```python
from build123d import *

# Parameters (mm, degrees)
SKETCH1_R           = 4.1275
BOSS_EXTRUDE2_DEPTH = 9.525
SKETCH3_R           = 6.35
CUT_EXTRUDE1_DEPTH  = 3.81
SKETCH4_W           = 33.423596482
SKETCH4_H           = 7.62
CUT_EXTRUDE3_DEPTH  = 53.073871807
FILLET3_R           = 0.8128
CHAMFER5_SIZE       = 0.8128


with BuildPart() as part:
    # Sketch1 → Boss-Extrude2 (new, symmetric)
    with BuildSketch(Plane.XY):
        with BuildLine():
            Line((0, 12.7), (31.75, 12.7))
            ThreePointArc((31.75, 12.7), (44.45, 0), (31.75, -12.7))
            Line((31.75, -12.7), (0, -12.7))
            ThreePointArc((0, -12.7), (-12.7, 0), (0, 12.7))
        make_face()
        with Locations(Location((0, 0, 0), (0, 0, 180))):
            Circle(SKETCH1_R, mode=Mode.SUBTRACT)
        with Locations(Location((31.75, 0, 0), (0, 0, 180))):
            Circle(SKETCH1_R, mode=Mode.SUBTRACT)
    extrude(amount=BOSS_EXTRUDE2_DEPTH, both=True)

    # Sketch3 → Cut-Extrude1 (cut)
    with BuildSketch(Plane.XY.offset(9.525)):
        Circle(SKETCH3_R)
        with Locations((31.75, 0)):
            Circle(SKETCH3_R)
    cut_extrude1 = extrude(amount=-CUT_EXTRUDE1_DEPTH, mode=Mode.SUBTRACT)

    # Mirror1: Cut-Extrude1 across plane
    add(cut_extrude1.mirror(Plane.XY), mode=Mode.SUBTRACT)

    # Sketch4 → Cut-Extrude3 (cut, through all)
    with BuildSketch(Plane(origin=(0, 12.7, 0), x_dir=(1, 0, 0), z_dir=(0, 1, 0))):
        with Locations((35.707937548, 0)):
            Rectangle(SKETCH4_W, SKETCH4_H)
        with Locations((-3.957937548, 0)):
            Rectangle(SKETCH4_W, SKETCH4_H)
    extrude(amount=-CUT_EXTRUDE3_DEPTH, mode=Mode.SUBTRACT)

    # Fillet3
    fillet3_edges = [part.edges().sort_by_distance(p)[0] for p in [
        (44.45, 0, 9.525),
        (15.875, 12.7, 9.525),
        (-12.7, 0, 9.525),
        (15.875, 12.7, -9.525),
        (25.373069653, 12.7, -3.81),
        (6.376930347, 12.7, 3.81),
        (44.45, 0, -9.525),
        (15.875, -12.7, -9.525),
        (-12.7, 0, -9.525),
        (6.376930347, -12.7, -3.81),
        (-12.7, 0, -3.81),
        (-12.7, 0, 3.81),
        (6.376930347, -12.7, 3.81),
        (12.753860693, -12.7, 0),
        (12.753860693, 12.7, 0),
        (6.376930347, 12.7, -3.81),
        (25.373069653, 12.7, 3.81),
        (18.996139307, 12.7, 0),
        (44.45, 0, -3.81),
        (25.373069653, -12.7, -3.81),
        (25.373069653, -12.7, 3.81),
        (44.45, 0, 3.81),
        (15.875, -12.7, 9.525),
        (18.996139307, -12.7, 0),
    ]]
    fillet(fillet3_edges, radius=FILLET3_R)

    # Chamfer5
    chamfer5_edges = [part.edges().sort_by_distance(p)[0] for p in [
        (4.1275, 0, 5.715),
        (-6.35, 0, 9.525),
        (35.8775, 0, 5.715),
        (25.4, 0, 9.525),
        (-6.35, 0, -9.525),
        (4.1275, 0, -5.715),
        (25.4, 0, -9.525),
        (35.8775, 0, -5.715),
        (4.1275, 0, -3.81),
        (4.1275, 0, 3.81),
        (35.8775, 0, -3.81),
        (35.8775, 0, 3.81),
    ]]
    chamfer(chamfer5_edges, length=CHAMFER5_SIZE)


solid = part.part
```
CAD build for the part. Positions are in the model's coordinates, mm. A direction names the side the tool comes from. Round coordinates to 2 decimals unless told otherwise and drop trailing zeros. Write each loop counter-clockwise with the first axis right and the second up, starting at its lowest first coordinate (ties: lowest second). Pieces come first, ordered by that corner, then holes. Notation, with made-up numbers: (50, -8) -> (66, -8) arc R26 cw to (66, 8) -> close; hole circle Ø8 at (30.5, -21). An arc over 180 degrees is marked (long way). Answer in a Markdown table with one row per item. Add a question column.
Item 1: Saw through at B-B, the plane z = 7.5. Write the cut outline in (x, y), then the cut area to 3 significant figures.
Item 2: Saw through at A-A, the plane x = 8. Write the cut outline in (y, z) (3 decimals), then the cut area to 3 significant figures.
Item 3: Mould opens along Z. For faces 4 (the face through (16, 0, -9.525)), 5 (the face through (12.754, 0, 0)), 6 (the face through (-12.697, -0.279, 6.696)), 7 (the face through (26, 0, -3.81)) say: pulls with the +Z half, pulls with the -Z half, needs draft (parallel to the pull), parting line crosses it, or undercut.
Item 4: Drop flat-ended pins along their axis: pin 1 Ø7.5 at (x, y) = (0, 0) entering from +Z; pin 2 Ø2 at (y, z) = (-5.5, 4.5) entering from -X; pin 3 Ø12 at (x, y) = (29.5, 5.5) entering from +Z (3 decimals); pin 4 Ø4 at (y, z) = (2, 1.5) entering from -X. Give the stop position or say it passes through.
Item 5: Which spindle directions (+Z, -Z, +X, -X, +Y, -Y) get a long thin tool onto all of the face, cutting with end or side? Do faces 1 (the face through (35, -4, -5.715)), 2 (the face through (6, 0, -3.81)), 3 (the face through (26, 0, 3.81)). Say none if no direction does.
Item 6: Saw through at C-C, the plane y = 2.75. Count the separate pieces of the cut face and the enclosed holes in it, then the cut area to 3 significant figures.
Item 7: Drill centre lines: line 1 (Z direction, x = 5, y = 1) (3 decimals); line 2 (Z direction, x = 40.5, y = 4) (3 decimals); line 3 (Y direction, x = 0, z = -4.75). Where is each one in solid material? Low to high. Write a range as from..to.
Findings below:
| question | item | result |
|---|---|---|
| 1 | outline | (0, -12.7) -> (31.75, -12.7) arc R12.7 ccw to (31.75, 12.7) -> (0, 12.7) arc R12.7 ccw to start; hole circle Ø12.7 at (0, 0); hole circle Ø12.7 at (31.75, 0) |
| 1 | area | 1,060 mm^2 |
| 2 | outline | (-12.7, -8.712) arc R0.813 ccw to (-11.887, -9.525) -> (11.887, -9.525) arc R0.813 ccw to (12.7, -8.712) -> (12.7, -4.623) arc R0.813 ccw to (11.887, -3.81) -> (-11.887, -3.81) arc R0.813 ccw to (-12.7, -4.623) -> close; (-12.7, 4.623) arc R0.813 ccw to (-11.887, 3.81) -> (11.887, 3.81) arc R0.813 ccw to (12.7, 4.623) -> (12.7, 8.712) arc R0.813 ccw to (11.887, 9.525) -> (-11.887, 9.525) arc R0.813 ccw to (-12.7, 8.712) -> close |
| 2 | area | 289 mm^2 |
| 3 | face 4 | pulls with the -Z half |
| 3 | face 5 | undercut |
| 3 | face 6 | needs draft |
| 3 | face 7 | undercut |
| 4 | pin 1 | passes through |
| 4 | pin 2 | stops at x = -11.87 |
| 4 | pin 3 | stops at z = 9.525 |
| 4 | pin 4 | stops at x = 12.75 |
| 5 | face 1 | -Z |
| 5 | face 2 | -X, +Y, -Y |
| 5 | face 3 | +X, +Y, -Y |
| 6 | separate pieces | 5 |
| 6 | enclosed holes | 0 |
| 6 | area | 462 mm^2 |
| 7 | line 1 | z = -5.715..-3.81, 3.81..5.715 |
| 7 | line 2 | z = -9.525..-3.81, 3.81..9.525 |
| 7 | line 3 | y = -12.7..-4.13, 4.13..12.7 |
